Read the model definition and answer for the solid it produces. Units are mm, in the model's axes. Round coordinates to 2 decimals unless told otherwise and drop trailing zeros. Loops run counter-clockwise (first coordinate to the right, second up) from the corner with the lowest first, then second, coordinate; pieces in that order, holes last. Notation, with made-up numbers: M -8.5,-10 L 7.5,-10 A25 ccw 7.5,23 Z; hole C -10.75,1.25 d2. An arc over 180 degrees is marked long. Write each question's results on one line, items separated by ' | '.
Autodesk Inventor part; units mm, degrees
ref_plane "YZ Plane" through (0, 0, 0) normal (1, 0, 0) x (0, 1, 0)
ref_plane "XZ Plane" through (0, 0, 0) normal (0, 1, 0) x (-1, 0, 0)
ref_plane "XY Plane" through (0, 0, 0) normal (0, 0, 1) x (1, 0, 0)
sketch "Sketch1" plane through (0, 0, 0) normal (0, 0, 1) x (1, 0, 0)
  line L0 (-55, 0) -> (55, 0) construction
  line L1 (-55, -10) -> (55, -10)
  line L2 (55, 10) -> (-55, 10)
  arc A0 (-55, 10) -> (-55, -10) centre (-55, 0) ccw
  arc A1 (55, -10) -> (55, 10) centre (55, 0) ccw
  circle A2 centre (-55, 0) radius 2.75
  circle A3 centre (55, 0) radius 2.75
  point P0 (0, 0)
  dimension "d0" = 10
  dimension "d1" = 110
  dimension "d2" = 5.5
extrude "Extrusion1" add sketch "Sketch1" along normal blind 1.1
sketch "Sketch2" plane through (0, 0, 1.1) normal (0, 0, 1) x (1, 0, 0)
  line L0 (42.5, 0) -> (-42.5, 0) construction
  line L1 (42.5, 2.75) -> (-42.5, 2.75)
  line L2 (-42.5, -2.75) -> (42.5, -2.75)
  arc A0 (42.5, -2.75) -> (42.5, 2.75) centre (42.5, 0) ccw
  arc A1 (-42.5, 2.75) -> (-42.5, -2.75) centre (-42.5, 0) ccw
  point P0 (0, 0)
  dimension "d5" = 5.5
  dimension "d6" = 85
extrude "Extrusion2" add sketch "Sketch2" along normal blind 5
properties part number "OldWankelBracket"
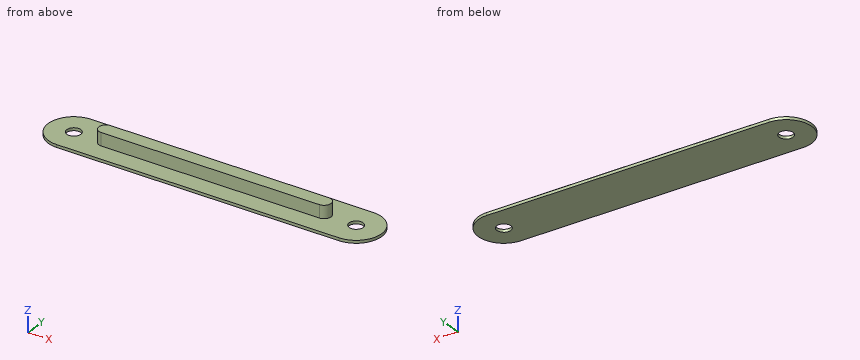
1. Given P1, Ø1.5, axis at x = 16, z = 2.5, coming from the -Y side; P2, Ø3, axis at x = -7, y = 6.5, coming from the +Z side, each flat-ended and moving along its own axis, determine where each tip first touches the part or whether it passes through.
Completed:
P1: stops at y = -2.75 | P2: stops at z = 1.1
2. Find section B-B, the plane y = -1.25. Give the vertices of the cut face in (x, z).
Completed:
outline: M -64.92,0 L -57.45,0 L -57.45,1.1 L -64.92,1.1 Z; M -52.55,0 L 52.55,0 L 52.55,1.1 L 44.95,1.1 L 44.95,6.1 L -44.95,6.1 L -44.95,1.1 L -52.55,1.1 Z; M 57.45,0 L 64.92,0 L 64.92,1.1 L 57.45,1.1 Z
3. Find the intervals of material crossed by L1, parallel to Y at x = -55, z = 0.95; L2, parallel to Y at x = -41, z = 2; L3, parallel to Z at x = -1, y = 5.75, in increasing order.
Completed:
L1: y = -10 to -2.75, 2.75 to 10 | L2: y = -2.75 to 2.75 | L3: z = 0 to 1.1
4. Find section D-D, the plane y = 8.25. Give the vertices of the cut face in (x, z), then the cut area to 3 significant figures.
Completed:
outline: M -60.65,0 L 60.65,0 L 60.65,1.1 L -60.65,1.1 Z | area: 133 mm2
5. Find section A-A, the plane x = -16. Give the vertices of the cut face in (y, z).
Completed:
outline: M -10,0 L 10,0 L 10,1.1 L 2.75,1.1 L 2.75,6.1 L -2.75,6.1 L -2.75,1.1 L -10,1.1 Z
6. Find section C-C, the plane z = 3.5. Give the vertices of the cut face in (x, y), then the cut area to 3 significant figures.
Completed:
outline: M -42.5,-2.75 L 42.5,-2.75 A2.75 ccw 42.5,2.75 L -42.5,2.75 A2.75 ccw Z | area: 491 mm2
